from build123d import *

# Parameters (mm, degrees)
SKETCH2_R           = 88.7
BOSS_EXTRUDE1_DEPTH = 24.7
BOSS_EXTRUDE2_START = 15
SKETCH3_R           = 88.7
SKETCH3_R_2         = 8.1375
BOSS_EXTRUDE2_DEPTH = 15
FILLET1_R           = 2
FILLET2_R           = 3
FILLET3_R           = 2


with BuildPart() as part:
    # Sketch2 → Boss-Extrude1 (new body)
    with BuildSketch(Plane.XY):
        with Locations((22.380830856, 278.150413141)):
            Circle(SKETCH2_R)
        with BuildLine():
            ThreePointArc((22.380830856, 354.550413141), (-54.019169144, 278.150413141), (22.380830856, 201.750413141))
            ThreePointArc((22.380830856, 201.750413141), (98.780830856, 278.150413141), (22.380830856, 354.550413141))
        make_face(mode=Mode.SUBTRACT)
    extrude(amount=-BOSS_EXTRUDE1_DEPTH)

    # Sketch3 → Boss-Extrude2 (add)
    with BuildSketch(Plane.XY.offset(BOSS_EXTRUDE2_START)):
        with Locations((22.380830856, 278.150413141)):
            Circle(SKETCH3_R)
        with Locations((12.834949907, 340.867975839)):
            Circle(SKETCH3_R_2, mode=Mode.SUBTRACT)
        with Locations((72.010243633, 317.73432135)):
            Circle(SKETCH3_R_2, mode=Mode.SUBTRACT)
        with Locations((-36.784620153, 301.21805109)):
            Circle(SKETCH3_R_2, mode=Mode.SUBTRACT)
        with Locations((-27.264784017, 238.487003795)):
            Circle(SKETCH3_R_2, mode=Mode.SUBTRACT)
        with Locations((31.880563493, 215.334967411)):
            Circle(SKETCH3_R_2, mode=Mode.SUBTRACT)
        with Locations((81.519347087, 254.971228106)):
            Circle(SKETCH3_R_2, mode=Mode.SUBTRACT)
        with BuildLine():
            ThreePointArc((61.996469473, 236.312741601), (54.216779809, 228.533051937), (61.996469473, 220.753362274))
            ThreePointArc((61.996469473, 220.753362274), (69.776159136, 228.533051937), (61.996469473, 236.312741601))
        make_face(mode=Mode.SUBTRACT)
    extrude(amount=-BOSS_EXTRUDE2_DEPTH)

    # Fillet1
    fillet1_edges = [part.edges().sort_by_distance(p)[0] for p in [
        (61.996469473, 220.753362274, 0),
    ]]
    fillet(fillet1_edges, radius=FILLET1_R)

    # Chamfer1: read off the stored shape, not the designer's step
    # Chamfer1 outline → Chamfer1 (revolve, cut)
    with BuildSketch(Plane(origin=(22.380830856, 278.150413141, 0), x_dir=(1, 0, 0), z_dir=(0, -1, 0))):
        Polygon((80.9, -24.7), (76.4, -16.7), (76.4, -24.7), align=None)
    revolve(axis=Axis((22.380830856, 278.150413141, 0), (0, 0, 1)), mode=Mode.SUBTRACT)

    # Fillet2
    fillet2_edges = [part.edges().sort_by_distance(p)[0] for p in [
        (76.403788939, 332.173371224, -16.7),
    ]]
    fillet(fillet2_edges, radius=FILLET2_R)

    # Fillet3
    fillet3_edges = [part.edges().sort_by_distance(p)[0] for p in [
        (-58.519169144, 278.150413141, -24.7),
    ]]
    fillet(fillet3_edges, radius=FILLET3_R)


solid = part.part
Read the model definition and answer for the solid it produces. Units are mm, in the model's axes. A direction names the side the tool comes from. Give positions to 0.01 mm unless a question says otherwise; leave off trailing zeros. Loops run counter-clockwise (first coordinate to the right, second up) from the corner with the lowest first, then second, coordinate; pieces in that order, holes last. Notation, with made-up numbers: (69, -19.5) - (101, -19.5) arc R23 ccw to (101, 6.5) - close; hole circle Ø1 at (2.5, 49.25). An arc over 180 degrees is marked (long way). Answer as CSV lines item,"result". Start each with the question number.
1) Which of the six approach directions +Z, -Z, +X, -X, +Y, -Y give full straight-line access (tool end or side, diameter ignored) to faces 5 (the face through (70.951, 325.803, 7.605)), 6 (the face through (-6.881, 207.576, -7.846))?
2) Find section C-C (z = 9). Write down the section's boundary in (x, y) (1 decimal), then the cut area to 3 significant figures.
3) Straight lines are drawn through the part: L1, parallel to Y at x = 86, z = 12.5; L2, parallel to Y at x = 80, z = -10.5; L3, parallel to X at y = 293.5, z = -16.5. For each, find the intervals that lie inside material, in ascending order. Write a range as from..to.
4) Find section A-A (z = -4). Write down the section's boundary in (x, y), then the cut area to 3 significant figures.
5) Determine the mould class of faces 1 (the face through (3.15, 191.56, -4.57)), 2 (the face through (79.755, 247.027, 7.605)), 3 (the face through (59.017, 221.347, 8.591)), 4 (the face through (101, 252, -24.7)) for opening direction X: released by +X, released by -X, zero draft, split by the parting line, or undercut.
6) Each of these flat-tipped pins is pushed along its axis until it touches: pin 1 Ø10 at (x, z) = (70.5, 6.5) entering from +Y; pin 2 Ø8 at (x, z) = (-29, 2) entering from +Y; pin 3 Ø8 at (x, z) = (86.5, -20) entering from -Y. Where does it stop, or does it pass through?
7) Find section B-B (y = 234). State how many separate pieces and enclosed holes the cut face has, then the cut area to 3 significant figures.
Findings below:
1,face 5,"+Z, -Z"
1,face 6,"-Z"
2,outline,"circle Ø177.4 at (22.4, 278.2); hole circle Ø16.3 at (-36.8, 301.2); hole circle Ø16.3 at (-27.3, 238.5); hole circle Ø16.3 at (12.8, 340.9); hole circle Ø16.3 at (31.9, 215.3); hole circle Ø15.6 at (62, 228.5); hole circle Ø16.3 at (72, 317.7); hole circle Ø16.3 at (81.5, 255)"
2,area,"23,300 mm^2"
3,L1,"216.34..248.18, 261.76..339.96"
3,L2,"210.71..227.98, 328.32..345.59"
3,L3,"-64.98..-52.52, 97.28..109.74"
4,outline,"circle Ø177.4 at (22.38, 278.15); hole circle Ø152.8 at (22.38, 278.15)"
4,area,"6,380 mm^2"
5,face 1,"split by the parting line"
5,face 2,"undercut"
5,face 3,"undercut"
5,face 4,"zero draft"
6,pin 1,"y = 355.66"
6,pin 2,"y = 353.14"
6,pin 3,"y = 212.93"
7,separate pieces,"3"
7,enclosed holes,"0"
7,area,"2,610 mm^2"
